CAD build for the part. Positions are in the model's coordinates, mm. A direction names the side the tool comes from. Round coordinates to 2 decimals unless told otherwise and drop trailing zeros. Loops run counter-clockwise (first coordinate to the right, second up) from the corner with the lowest first, then second, coordinate; pieces in that order, holes last.
from build123d import *


# Read off the part's stored shape, not the designer's step: Vaciado1
with BuildPart() as part:
    # Croquis1 → Revolución2 (revolve)
    with BuildSketch(Plane(origin=(0, 0, 0), x_dir=(1, 0, 0), z_dir=(0, 1, 0)), mode=Mode.PRIVATE) as revoluci_n2_sk:
        Polygon((0, -60), (0, 60), (-5, 60), (-5, 50), (-83, -60), (-88, -60), (-88, -62.5), (0, -62.5), align=None)
    revolve(revoluci_n2_sk.sketch.rotate(Axis((0, 0, 60), (0, 0, -1)), 180), axis=Axis((0, 0, 60), (0, 0, -1)))

    # Vaciado1 outline → Vaciado1 (revolve, cut)
    with BuildSketch(Plane.XZ):
        Polygon((0, -60), (2.5, -60), (2.5, -49.203587736), (81.707998576, 62.5), (0, 62.5), align=None)
    revolve(axis=Axis((0, 0, 0), (0, 0, 1)), mode=Mode.SUBTRACT)


solid = part.part
Item 1: Cut at B-B (z = 31). List the corners of the cut face in (x, y), plus the area to 3 significant figures.
Verdict:
outline: circle Ø124.87 at (0, 0); hole circle Ø118.74 at (0, 0)
area: 1,170 mm2
Item 2: Cut at A-A (x = 0). List the corners of the cut face in (y, z).
Verdict:
outline: (-88, 60) - (-83, 60) - (-5, -50) - (-5, -60) - (-2.5, -60) - (-2.5, -49.2) - (-81.71, 62.5) - (-88, 62.5) - close; (2.5, -60) - (5, -60) - (5, -50) - (83, 60) - (88, 60) - (88, 62.5) - (81.71, 62.5) - (2.5, -49.2) - close
Item 3: Wall check: L1, parallel to Y at x = 0, z = -55.25; L2, parallel to Y at x = 35, z = 57.5; L3, parallel to Z at x = 20, y = -9. Give the ranges that are in metal, low to high.
Verdict:
L1: y = -5 to -2.5, 2.5 to 5
L2: y = -73.3 to -69.89, 69.89 to 73.3
L3: z = -26.12 to -21.8
Item 4: Mould opens along X. For faces 3 (the cylindrical face through (-0.54, -2.44, -54.53)), 4 (the cylindrical face through (-5, 0, -55)), 5 (the flat face through (26, 78, 62.5)) say: released by +X, released by -X, zero draft, split by the parting line, or undercut.
Verdict:
face 3: undercut
face 4: split by the parting line
face 5: zero draft
Item 5: Flat gauge pins, fed straight in: P1, Ø5, axis at x = -57, y = -16.5, coming from the +Z side; P2, Ø5, axis at x = -58.5, y = -36, coming from the +Z side; P3, Ø10, axis at x = -61.5, y = 26.5, coming from the +Z side. Where does each tip first touch, or does it go through?
Verdict:
P1: stops at z = 34.48
P2: stops at z = 47.67
P3: stops at z = 48.76
Item 6: 3-axis set-ups, long thin cutter, end or side, ignore diameter. For faces 1 (the flat face through (53, 65, 60)), 2 (the cylindrical face through (-19.077, 85.907, 61.268)): which of +Z, -Z, +X, -X, +Y, -Y reach the whole face in a straight line?
Verdict:
face 1: -Z
face 2: +Z, -Z
Item 7: Cut at C-C (z = -16). List the corners of the cut face in (x, y), plus the area to 3 significant figures.
Verdict:
outline: circle Ø58.22 at (0, 0); hole circle Ø52.09 at (0, 0)
area: 531 mm2
